```python
from build123d import *

# Parameters (mm, degrees)
F0_R     = 50.8
F0_W     = 34.925
F0_H     = 34.925
F1_DEPTH = 25.4


with BuildPart() as f1:
    # F0 (on Front) → F1 (new body)
    with BuildSketch(Plane.XZ):
        Circle(F0_R)
        Rectangle(F0_W, F0_H, mode=Mode.SUBTRACT)
    extrude(amount=F1_DEPTH)


solid = f1.part
```
Geometry check sheet. Reference: the model listing, model coordinates, mm. A direction names the side the tool comes from. Give positions to 0.01 mm unless a question says otherwise; leave off trailing zeros. Write each loop counter-clockwise with the first axis right and the second up, starting at its lowest first coordinate (ties: lowest second). Pieces come first, ordered by that corner, then holes. Notation, with made-up numbers: (76.25, 20) - (126.25, 20) arc R19 ccw to (126.25, 35) - close; hole circle Ø5 at (62.25, -33). An arc over 180 degrees is marked (long way). Use a Markdown table: item, result.
Q1. Set-up check for faces 4 (the face through (-17.462, -13, 0)), 5 (the face through (22, 0, 1)): record each of +Z, -Z, +X, -X, +Y, -Y from which the full face is reachable in a straight line by a thin tool's end or side.
Computed:
| item | result |
|---|---|
| face 4 | +Y, -Y |
| face 5 | +Z, -Z, +X, -X, +Y |
Q2. Section check C-C, the plane y = -6.25. Enter the section's corners in (x, z).
Computed:
| item | result |
|---|---|
| outline | circle Ø101.6 at (0, 0); hole (-17.46, -17.46) - (17.46, -17.46) - (17.46, 17.46) - (-17.46, 17.46) - close |
Q3. Draft check along X on faces 1 (the face through (22, -25.4, 1)), 2 (the face through (17.462, -13, 0)), 3 (the face through (-11.012, -12.522, -49.592)). Enter one of: pulls with the +X half, pulls with the -X half, needs draft (parallel to the pull), parting line crosses it, or undercut.
Computed:
| item | result |
|---|---|
| face 1 | needs draft |
| face 2 | undercut |
| face 3 | parting line crosses it |
Q4. Section check A-A, the plane x = 0. Enter the section's corners in (y, z), then the cut area to 3 significant figures.
Computed:
| item | result |
|---|---|
| outline | (-25.4, -50.8) - (0, -50.8) - (0, -17.46) - (-25.4, -17.46) - close; (-25.4, 17.46) - (0, 17.46) - (0, 50.8) - (-25.4, 50.8) - close |
| area | 1,690 mm² |
Q5. Section check D-D, the plane x = 31. Enter the section's corners in (y, z), then the cut area to 3 significant figures.
Computed:
| item | result |
|---|---|
| outline | (-25.4, -40.24) - (0, -40.24) - (0, 40.24) - (-25.4, 40.24) - close |
| area | 2,040 mm² |
Q6. Thickness scan on L1, parallel to Z at x = 13.5, y = -8.25; L2, parallel to Z at x = 15.5, y = -12.25. Record the ranges inside material, lowest first. Write a range as [from, to].
Computed:
| item | result |
|---|---|
| L1 | z = [-48.97, -17.46], [17.46, 48.97] |
| L2 | z = [-48.38, -17.46], [17.46, 48.38] |
Q7. Section check B-B, the plane z = 0. Enter the section's corners in (x, y).
Computed:
| item | result |
|---|---|
| outline | (-50.8, -25.4) - (-17.46, -25.4) - (-17.46, 0) - (-50.8, 0) - close; (17.46, -25.4) - (50.8, -25.4) - (50.8, 0) - (17.46, 0) - close |
Q8. Go/stop test with flat-tipped pins: P1, Ø8, axis at x = -39.5, y = -20.5, coming from the +Z side; P2, Ø5, axis at y = -9.5, z = -39.5, coming from the +X side; P3, Ø4, axis at x = 5, z = -19.5, coming from the +Y side; P4, Ø2, axis at x = -22.5, y = -17, coming from the -Z side. Record where each tip stops, or that it passes through.
Computed:
| item | result |
|---|---|
| P1 | stops at z = 36.34 |
| P2 | stops at x = 34.81 |
| P3 | stops at y = 0 |
| P4 | stops at z = -46.03 |
